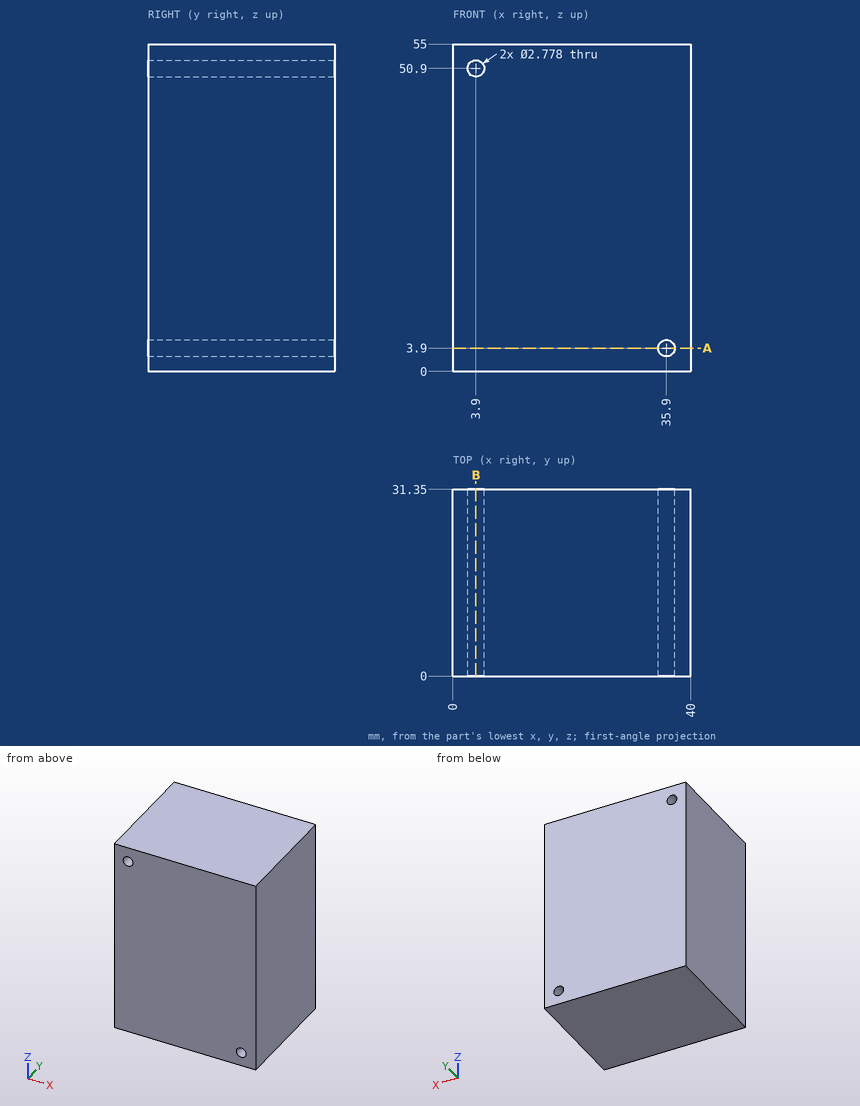
Can you work these out from the drawing? Everything is in mm from the part's minimum corner. Coordinates: 2 decimals unless noted, no trailing zeros. Write each loop counter-clockwise with the first axis right and the second up, starting at its lowest first coordinate (ties: lowest second). Pieces come first, ordered by that corner, then holes. Notation, with made-up numbers: (67.25, -5) -> (90.25, -5) arc R13 cw to (90.25, 8) -> close; hole circle Ø1 at (25.5, 8.25). An arc over 180 degrees is marked (long way). Write each question's results on one line, items separated by ' | '. Start each with the question number.
Item 1: If we section it at A-A, the plane z = 3.9: Write out the boundary of the cut face in (x, y).
Item 2: Please list where these lines run through material, in increasing order: probe 1 along Z at (x, y) = (3.9, 8.5); probe 2 along X at (y, z) = (25, 4) (1 decimal); probe 3 along Z at (x, y) = (3, 18).
Item 3: I'm going to push a flat-ended pin straight in: P1, Ø2, axis at x = 3.9, z = 50.9, coming from the -Y side. Where does the tip first touch, or does it pass through?
Item 4: If we section it at B-B, the plane x = 3.9: Write out the boundary of the cut face in (y, z).
Answer block:
1) outline: (0, 0) -> (34.51, 0) -> (34.51, 31.35) -> (0, 31.35) -> close; (37.29, 0) -> (40, 0) -> (40, 31.35) -> (37.29, 31.35) -> close
2) probe 1: 0 to 49.51, 52.29 to 55 | probe 2: 0 to 34.5, 37.3 to 40 | probe 3: 0 to 49.84, 51.96 to 55
3) P1: through
4) outline: (0, 0) -> (31.35, 0) -> (31.35, 49.51) -> (0, 49.51) -> close; (0, 52.29) -> (31.35, 52.29) -> (31.35, 55) -> (0, 55) -> close
